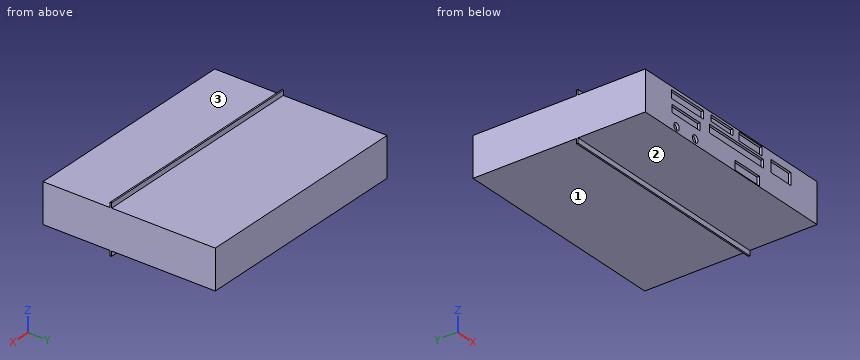
from build123d import *

# Parameters (mm, degrees)
F0_W     = 91
F0_H     = 16
F1_DEPTH = 70
F2_R     = 1.456775
F2_W     = 10.683106
F2_H     = 4.879937
F2_W_2   = 13.057131
F2_H_2   = 3.692926
F2_W_3   = 17.013836
F2_H_3   = 3.297256
F2_W_4   = 14.903594
F2_H_4   = 3.033476
F2_W_5   = 11.60634
F2_H_5   = 2.505915
F2_W_6   = 12.00201
F2_H_6   = 3.429146
F2_W_7   = 28.620178
F2_H_7   = 3.297255
F3_DEPTH = 1
F4_W     = 0.6
F4_H     = 2
F5_DEPTH = 91


with BuildPart() as f1:
    # F0 (on Front) → F1 (new body)
    with BuildSketch(Plane.XZ):
        Rectangle(F0_W, F0_H)
    extrude(amount=-F1_DEPTH)

    # F2 (on face) → F3 (cut)
    with BuildSketch(Plane.XZ):
        with Locations((-28.951265, -5.898637)):
            Circle(F2_R)
        with Locations((-19.059498, -5.898637)):
            Circle(F2_R)
        with Locations((26.376682, 2.608282)):
            Rectangle(F2_W, F2_H)
        with Locations((8.571502, -5.898637)):
            Rectangle(F2_W_2, F2_H_2)
        with Locations((-23.08215, 5.114197)):
            Rectangle(F2_W_3, F2_H_3)
        with Locations((-24.005381, -0.161412)):
            Rectangle(F2_W_4, F2_H_4)
        with Locations((-4.947245, 5.773649)):
            Rectangle(F2_W_5, F2_H_5)
        with Locations((10.286076, 5.839593)):
            Rectangle(F2_W_6, F2_H_6)
        with Locations((2.768333, 1.55316)):
            Rectangle(F2_W_7, F2_H_7)
    extrude(amount=-F3_DEPTH, mode=Mode.SUBTRACT)

    # F4 (on face) → F5 (join, through all)
    with BuildSketch(Plane.YZ.offset(45.5)):
        with Locations((27.6, 9)):
            Rectangle(F4_W, F4_H)
        with Locations((27.6, -9)):
            Rectangle(F4_W, F4_H)
    extrude(amount=-F5_DEPTH)


solid = f1.part
Verification items for the finished model (mm, model axes). Face numbers are marked on the shaded views. A direction names the side the tool comes from. Give positions to 0.01 mm unless a question says otherwise; leave off trailing zeros. Order: outer loops, then holes, each group sorted by start corner. A loop starts at its lowest first (then second) coordinate and runs counter-clockwise, first axis right, second up. Notation, with made-up numbers: M 28.5,22.5 L 87.5,22.5 A25 ccw 87.5,45.5 Z; hole C 10.25,65 d10. An arc over 180 degrees is marked long. Answer as a JSON object with one key per item and string values. Group by question number.
1) Cross-section at A-A (x = -6). Enter the section's corners in (y, z).
2) Depth check by flat-ended pin: pin 1 Ø8 at (x, y) = (1.5, 18) entering from -Z; pin 2 Ø4 at (x, y) = (-8.5, 27) entering from -Z; pin 3 Ø0.6 at (x, z) = (-12.5, -9) entering from -Y; pin 4 Ø10 at (x, y) = (30, 56.5) entering from +Z. Enter the tip coordinate at first touch or a pass-through.
3) Cross-section at C-C (x = 23.5). Enter the section's corners in (y, z).
4) Scan lines: line 1 along Z through (x, y) = (0.5, 19.5); line 2 along Y through (x, z) = (23, 1.25). Record each from-to range of solid material in increasing order. Write a range as [from, to].
5) Cross-section at B-B (y = 12.5). Enter the section's corners in (x, z).
6) Cross-section at D-D (x = -40). Enter the section's corners in (y, z), then the cut area to 3 significant figures.
7) Access from +Z, -Z, +X, -X, +Y, -Y to the whole of each face (thin tool, end or side, straight path). Record for the marked faces 1, 2 and 3.
Result sheet:
{
 "1": {"outline": "M 0,-8 L 27.3,-8 L 27.3,-10 L 27.9,-10 L 27.9,-8 L 70,-8 L 70,8 L 27.9,8 L 27.9,10 L 27.3,10 L 27.3,8 L 0,8 L 0,7.03 L 1,7.03 L 1,4.52 L 0,4.52 L 0,3.2 L 1,3.2 L 1,-0.1 L 0,-0.1 Z"},
 "2": {"pin 1": "stops at z = -8", "pin 2": "stops at z = -10", "pin 3": "stops at y = 27.3", "pin 4": "stops at z = 8"},
 "3": {"outline": "M 0,-8 L 27.3,-8 L 27.3,-10 L 27.9,-10 L 27.9,-8 L 70,-8 L 70,8 L 27.9,8 L 27.9,10 L 27.3,10 L 27.3,8 L 0,8 L 0,5.05 L 1,5.05 L 1,0.17 L 0,0.17 Z"},
 "4": {"line 1": "z = [-8, 8]", "line 2": "y = [1, 70]"},
 "5": {"outline": "M -45.5,-8 L 45.5,-8 L 45.5,8 L -45.5,8 Z"},
 "6": {"outline": "M 0,-8 L 27.3,-8 L 27.3,-10 L 27.9,-10 L 27.9,-8 L 70,-8 L 70,8 L 27.9,8 L 27.9,10 L 27.3,10 L 27.3,8 L 0,8 Z", "area": "1,120 mm2"},
 "7": {"face 1": "-Z, +X, -X, +Y", "face 2": "-Z, +X, -X, -Y", "face 3": "+Z, +X, -X, -Y"}
}
